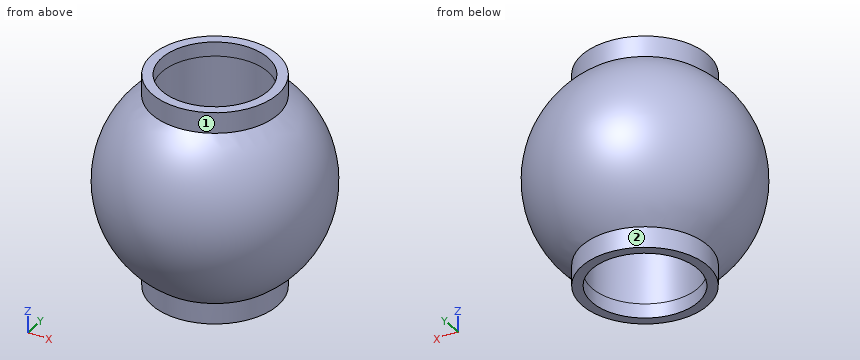
from build123d import *

# Parameters (mm, degrees)
ENL_V_MAT_EXTRU_1_DEPTH      = 6.196152423
ENL_V_MAT_EXTRU_1_DEPTH_BACK = 6.196152423
ESQUISSE2_R                  = 1.5
BOSS_EXTRU_1_DEPTH           = 3
BOSS_EXTRU_1_DEPTH_BACK      = 3
ESQUISSE3_R                  = 1.776748734
ESQUISSE3_R_2                = 1.5


with BuildPart() as part:
    # Esquisse1 → Révolution1 (revolve)
    with BuildSketch(Plane.XY):
        with BuildLine():
            Line((0, -3), (0, 3))
            ThreePointArc((0, 3), (-3, 0), (0, -3))
        make_face()
    revolve(axis=Axis((0, 4.208011384, 0), (0, -1, 0)))

    # Esquisse2 → Enlèv. mat.-Extru.1 (cut, two sides: drawn at the far end of the back side and taken through both)
    with BuildSketch(Plane.XY.offset(-ENL_V_MAT_EXTRU_1_DEPTH_BACK)):
        Circle(ESQUISSE2_R)
    extrude(amount=ENL_V_MAT_EXTRU_1_DEPTH + ENL_V_MAT_EXTRU_1_DEPTH_BACK, mode=Mode.SUBTRACT)

    # Esquisse3 → Boss.-Extru.1 (add, two sides: drawn at the far end of the back side and taken through both)
    with BuildSketch(Plane.XY.offset(-BOSS_EXTRU_1_DEPTH_BACK)):
        Circle(ESQUISSE3_R)
        Circle(ESQUISSE3_R_2, mode=Mode.SUBTRACT)
    extrude(amount=BOSS_EXTRU_1_DEPTH + BOSS_EXTRU_1_DEPTH_BACK)


solid = part.part
Can you work these out from the model? Positions are in its coordinate system, mm. Face numbers are marked on the shaded views. A direction names the side the tool comes from. Coordinates: 2 decimals unless noted, no trailing zeros. Loops run counter-clockwise (first coordinate to the right, second up) from the corner with the lowest first, then second, coordinate; pieces in that order, holes last. Notation, with made-up numbers: (-14.5, -27) - (22.5, -27) arc R7 ccw to (22.5, -21) - close; hole circle Ø5 at (36, 72.25). An arc over 180 degrees is marked (long way). Answer as a JSON object with one key per item and string values. Group by question number.
Item 1: For pin 1 (1.5 mm diameter, centred on x = 1, z = -1.5, fed in from +Y); pin 2 (2 mm diameter, centred on y = 1, z = 0.5, fed in from +X); pin 3 (2 mm diameter, centred on x = 2, z = 0.5, fed in from -Y), each with a flat end and sliding along its axis, tell me the tip position at first contact or that it passes through.
Item 2: If we section it at A-A (x = 0): List the corners of the cut face in (y, z) for me, plus the area to 3 significant figures.
Item 3: On a 3-axis mill with a long thin cutter (end or side, diameter ignored), from which of +Z, -Z, +X, -X, +Y, -Y can I reach the whole of each face in a straight line? I mean the marked faces 1 and 2. Say none if no direction works.
Item 4: If we section it at C-C (z = -1.5): List the corners of the cut face in (x, y) for me, plus the area to 3 significant figures.
Item 5: If we section it at D-D (y = -2.4): List the corners of the cut face in (x, z) for me, plus the area to 3 significant figures.
Item 6: If I drill on L1, parallel to X at y = 0, z = -2.7; L2, parallel to Y at x = 0, z = 1.1, over which ranges is the centre line in solid material (lowest first)? Write a range as from..to.
Returned:
{
 "1": {"pin 1": "stops at y = 2.81", "pin 2": "stops at x = 3", "pin 3": "stops at y = -2.81"},
 "2": {"outline": "(-1.78, -3) - (-1.5, -3) - (-1.5, 3) - (-1.78, 3) - (-1.78, 2.42) arc R3 ccw to (-1.78, -2.42) - close; (1.5, -3) - (1.78, -3) - (1.78, -2.42) arc R3 ccw to (1.78, 2.42) - (1.78, 3) - (1.5, 3) - close", "area": "11.6 mm²"},
 "3": {"face 1": "+Z", "face 2": "-Z"},
 "4": {"outline": "circle Ø5.2 at (0, 0); hole circle Ø3 at (0, 0)", "area": "14.1 mm²"},
 "5": {"outline": "circle Ø3.6 at (0, 0)", "area": "10.2 mm²"},
 "6": {"L1": "x = -1.78..-1.5, 1.5..1.78", "L2": "y = -2.79..-1.5, 1.5..2.79"}
}
